Can you work these out from the model? Positions are in its coordinate system, mm. Face numbers are marked on the shaded views. A direction names the side the tool comes from. Coordinates: 2 decimals unless noted, no trailing zeros. Order: outer loops, then holes, each group sorted by start corner. A loop starts at its lowest first (then second) coordinate and runs counter-clockwise, first axis right, second up. Notation, with made-up numbers: (-16.5, -4.75) - (27.5, -4.75) arc R11 ccw to (27.5, 15.25) - close; hole circle Ø9 at (86, 71.25). An arc over 180 degrees is marked (long way). Use a Markdown table: item, result. Add a question column.
(1) I want a section at C-C (y = 55). List the corners of the cut face in (x, z) for me.
(2) I want a section at B-B (z = -0.75). List the corners of the cut face in (x, y) for me, and give its area (3 significant figures).
(3) If I drill on L1, parallel to Y at x = 199, z = -0.75; L2, parallel to X at y = 56.5, z = 1.75; L3, parallel to X at y = 8, z = 1.25, over which ranges is the centre line in solid material (lowest first)? Write a range as [from, to].
(4) On a 3-axis mill with a long thin cutter (end or side, diameter ignored), from which of +Z, -Z, +X, -X, +Y, -Y can I reach the whole of each face in a straight line? I mean the marked faces 1 and 2. Say none if no direction works.
(5) I want a section at A-A (x = 203). List the corners of the cut face in (y, z) for me, and give its area (3 significant figures).
(6) I want a section at D-D (x = 197). List the corners of the cut face in (y, z) for me, and give its area (3 significant figures).
(7) For pin 1 Ø1 at (x, y) = (205.5, 27.5) entering from -Z; pin 2 Ø1.5 at (x, z) = (208.5, 5.5) entering from -Y; pin 3 Ø5 at (y, z) = (50, 0.5) entering from -X; pin 4 Ø1.5 at (y, z) = (8.5, 1) entering from +X, each with a flat end and sliding along its axis, tell me the tip position at first contact or that it passes through.
```python
from build123d import *

# Parameters (mm, degrees)
CYLINDER032_R             = 4
CYLINDER032_DEPTH         = 70
PRISM004_DEPTH            = 6
FUSION014_PLACEMENT_ANGLE = 90


with BuildPart() as cilindro032:
    # Cylinder032 → Cylinder032 (new body)
    with BuildSketch(Plane.XY):
        Circle(CYLINDER032_R)
    extrude(amount=CYLINDER032_DEPTH)


with BuildPart() as tornillo_m8:
    # Prism004 → Prism004 (new body)
    with BuildSketch(Plane.XY):
        Polygon((7.19, 0), (3.595, 6.226723), (-3.595, 6.226723), (-7.19, 0), (-3.595, -6.226723), (3.595, -6.226723), align=None)
    extrude(amount=PRISM004_DEPTH)

    # Fusion014: union Cilindro032
    add(cilindro032.part)


with BuildPart() as tornillo_m8_1:
    # Fusion014 placement: moved
    add(tornillo_m8.part.moved(Location((203, -3, 2))).rotate(Axis((203, -3, 2), (-1, 0, 0)), FUSION014_PLACEMENT_ANGLE))


solid = tornillo_m8_1.part
```
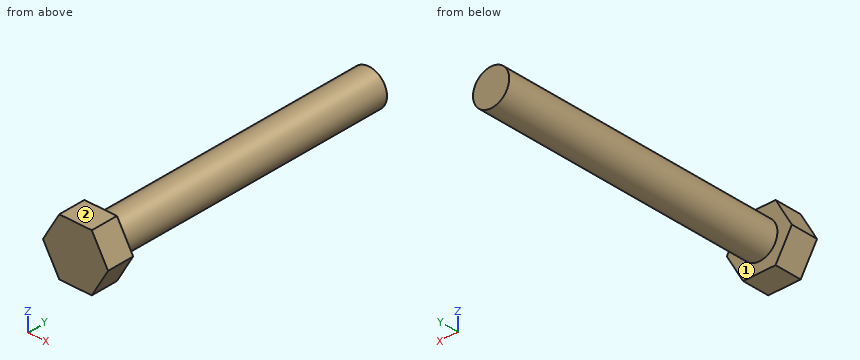
Answers follow:
| question | item | result |
|---|---|---|
| 1 | outline | circle Ø8 at (203, 2) |
| 2 | outline | (197.4, -3) - (208.6, -3) - (208.6, 3) - (205.9, 3) - (205.9, 67) - (200.1, 67) - (200.1, 3) - (197.4, 3) - close |
| 2 | area | 439 mm² |
| 3 | L1 | y = [-3, 3] |
| 3 | L2 | x = [199.01, 206.99] |
| 3 | L3 | x = [199.07, 206.93] |
| 4 | face 1 | +Y |
| 4 | face 2 | +Z, +X, -X, +Y, -Y |
| 5 | outline | (-3, -4.23) - (3, -4.23) - (3, -2) - (67, -2) - (67, 6) - (3, 6) - (3, 8.23) - (-3, 8.23) - close |
| 5 | area | 587 mm² |
| 6 | outline | (-3, -0.06) - (3, -0.06) - (3, 4.06) - (-3, 4.06) - close |
| 6 | area | 24.7 mm² |
| 7 | pin 1 | stops at z = -1.46 |
| 7 | pin 2 | stops at y = -3 |
| 7 | pin 3 | stops at x = 199 |
| 7 | pin 4 | stops at x = 206.99 |
